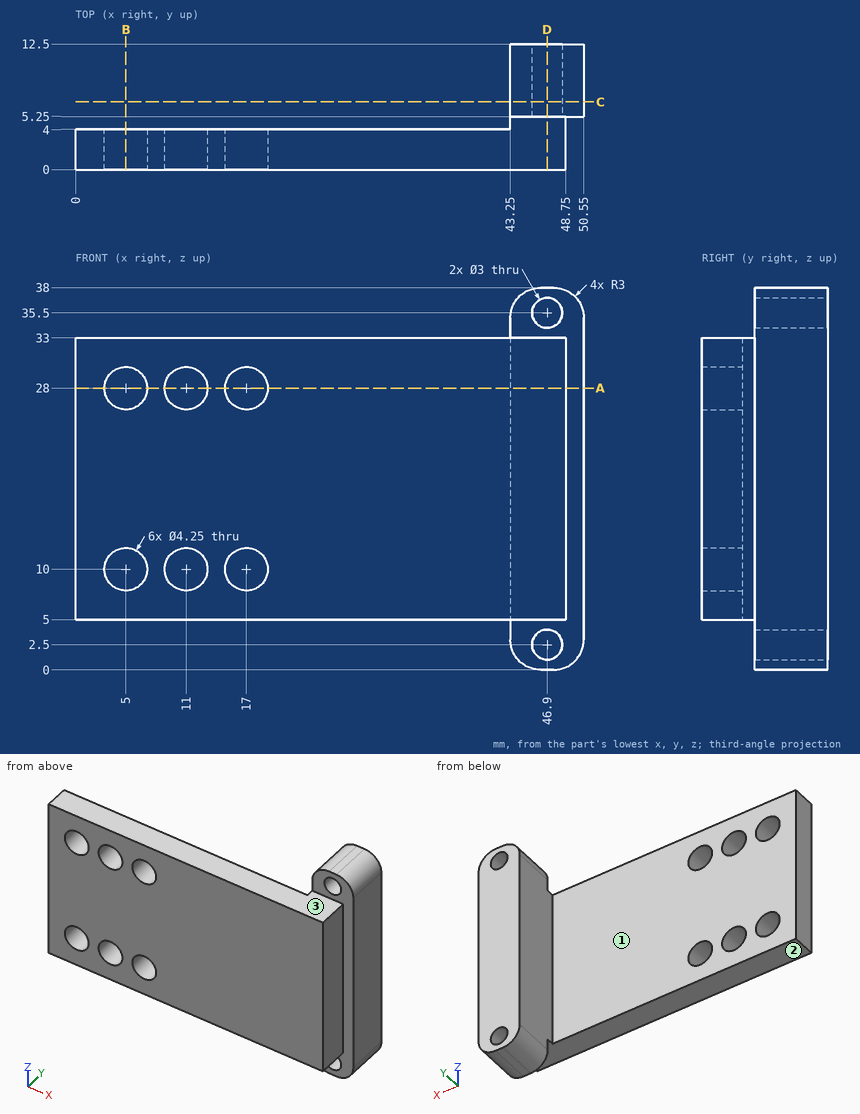
Could you check a few things on this drawing? It's one solid part, dimensions in mm from its lowest x, y, z. A direction names the side the tool comes from. Coordinates: 2 decimals unless noted, no trailing zeros. Order: outer loops, then holes, each group sorted by start corner. A loop starts at its lowest first (then second) coordinate and runs counter-clockwise, first axis right, second up. Notation, with made-up numbers: (-28, 75) -> (8, 75) arc R22 ccw to (8, 108) -> close; hole circle Ø4 at (22, 27). An arc over 180 degrees is marked (long way). One line per item, written item: value. Start each with the question number.
1) Which directions (+Z, -Z, +X, -X, +Y, -Y) give clear straight access to the entire face, cutting with the end or side of a thin tool? Please do the marked faces 1, 2 and 3.
2) Imagine slicing it at A-A on z = 28. List the corners of the cut face in (x, y) for me (3 decimals), plus the area to 3 significant figures.
3) Imagine slicing it at C-C on y = 6.75. List the corners of the cut face in (x, z) for me, plus the area to 3 significant figures.
4) Imagine slicing it at D-D on x = 46.9. List the corners of the cut face in (y, z) for me, plus the area to 3 significant figures.
5) Imagine slicing it at B-B on x = 5. List the corners of the cut face in (y, z) for me (3 decimals), plus the area to 3 significant figures.
6) I'm going to push flat-ended pins straight in: pin 1 (2.5 mm diameter, centred on x = 20, y = 3.5, fed in from -Z); pin 2 (3.5 mm diameter, centred on x = 46.9, z = 2.5, fed in from -Y); pin 3 (8 mm diameter, centred on x = 18, z = 19.5, fed in from +Y). Where does each tip first touch, or does it pass through?
7) If I drill on L1, parallel to X at y = 1.25, z = 10 (3 decimals); L2, parallel to Z at x = 5, y = 3.1 (3 decimals); L3, parallel to Z at x = 46.9, y = 9.5, over which ranges is the centre line in solid material (lowest first)? Write a range as [from, to].
Answer list:
1. face 1: +Z, -Z, -X, +Y
1. face 2: -Z, +X, -X, -Y
1. face 3: +Z, +X, -X, -Y
2. outline: (0, 0) -> (2.875, 0) -> (2.875, 4) -> (0, 4) -> close; (7.125, 0) -> (8.875, 0) -> (8.875, 4) -> (7.125, 4) -> close; (13.125, 0) -> (14.875, 0) -> (14.875, 4) -> (13.125, 4) -> close; (19.125, 0) -> (48.75, 0) -> (48.75, 5.25) -> (50.55, 5.25) -> (50.55, 12.5) -> (43.25, 12.5) -> (43.25, 4) -> (19.125, 4) -> close
2. area: 204 mm2
3. outline: (43.25, 3) arc R3 ccw to (46.25, 0) -> (47.55, 0) arc R3 ccw to (50.55, 3) -> (50.55, 35) arc R3 ccw to (47.55, 38) -> (46.25, 38) arc R3 ccw to (43.25, 35) -> close; hole circle Ø3 at (46.9, 2.5); hole circle Ø3 at (46.9, 35.5)
3. area: 256 mm2
4. outline: (0, 5) -> (5.25, 5) -> (5.25, 4) -> (12.5, 4) -> (12.5, 34) -> (5.25, 34) -> (5.25, 33) -> (0, 33) -> close; (5.25, 0) -> (12.5, 0) -> (12.5, 1) -> (5.25, 1) -> close; (5.25, 37) -> (12.5, 37) -> (12.5, 38) -> (5.25, 38) -> close
4. area: 379 mm2
5. outline: (0, 5) -> (4, 5) -> (4, 7.875) -> (0, 7.875) -> close; (0, 12.125) -> (4, 12.125) -> (4, 25.875) -> (0, 25.875) -> close; (0, 30.125) -> (4, 30.125) -> (4, 33) -> (0, 33) -> close
5. area: 78.0 mm2
6. pin 1: stops at z = 5
6. pin 2: stops at y = 5.25
6. pin 3: stops at y = 4
7. L1: x = [0, 2.875], [7.125, 8.875], [13.125, 14.875], [19.125, 48.75]
7. L2: z = [5, 7.875], [12.125, 25.875], [30.125, 33]
7. L3: z = [0, 1], [4, 34], [37, 38]
